```python
from build123d import *

# Parameters (mm, degrees)
F0_W        = 77.47
F0_H        = 19.05
F0_R        = 1.3890625
F0_W_2      = 52.07
F0_H_2      = 8.255
F0_W_3      = 7.62
F1_DEPTH    = 2.0574
F2_R        = 1.3890625
F2_W        = 46.99
F2_H        = 20.1539304107
F3_DEPTH    = 25.4
F4_T1_DEPTH = 2.0574


# Not quite as in the source:
# - a fillet or chamfer that OpenCascade refuses, or shapes differently, is made with other operations: its cross-section is extruded or revolved along the edge and cut away or added


with BuildPart() as f1:
    # F0 (on Top) → F1 (new body)
    with BuildSketch(Plane.XY):
        with Locations((29.845, 0)):
            Rectangle(F0_W, F0_H)
        with Locations((-4.2449974041, 0)):
            Circle(F0_R, mode=Mode.SUBTRACT)
        with Locations((-34.925, -13.6525)):
            Rectangle(F0_W_2, F0_H_2)
        with Locations((-34.925, 0)):
            Rectangle(F0_W_2, F0_H)
        with Locations((-64.77, 0)):
            Rectangle(F0_W_3, F0_H)
        with Locations((-64.6969974041, 0)):
            Circle(F0_R, mode=Mode.SUBTRACT)
        with Locations((-34.925, 13.6525)):
            Rectangle(F0_W_2, F0_H_2)
    extrude(amount=F1_DEPTH)

    # F2 (on face) → F3 (cut)
    with BuildSketch(Plane.XY.offset(2.0574)):
        Polygon((43.5640997417, 9.525), (68.58, 4.0749409236), (68.58, 9.525), align=None)
        Polygon((68.58, -9.525), (68.58, -4.0749409236), (43.5640997417, -9.525), align=None)
        with Locations((49.53, 0)):
            Circle(F2_R)
        with Locations((62.23, 0)):
            Circle(F2_R)
        with Locations((-35.5063436133, 0.5281241611)):
            Rectangle(F2_W, F2_H)
    extrude(amount=-F3_DEPTH, mode=Mode.SUBTRACT)

    # F4: fillet of radius 10.16 on 4 edges, made by hand

    # F4_s2 → F4_t1 (join)
    with BuildSketch(Plane.XY):
        with BuildLine():
            add(Edge.make_bspline(
                [(-22.1713436133, 10.6050893664), (-12.0113436133, 10.6050893664), (-12.0113436133, 0.4450893664)],
                knots=[0, 0, 0, 1, 1, 1], degree=2, weights=[1, 2.3333333333, 1]))
            Line((-12.0113436133, 0.4450893664), (-12.0113436133, 10.6050893664))
            Line((-12.0113436133, 10.6050893664), (-22.1713436133, 10.6050893664))
        make_face()
        with BuildLine():
            add(Edge.make_bspline(
                [(-48.8413436133, 10.6050893664), (-59.0013436133, 10.6050893664), (-59.0013436133, 0.4450893664)],
                knots=[0, 0, 0, 1, 1, 1], degree=2, weights=[1, 2.3333333333, 1]))
            Line((-59.0013436133, 0.4450893664), (-59.0013436133, 10.6050893664))
            Line((-59.0013436133, 10.6050893664), (-48.8413436133, 10.6050893664))
        make_face()
        with BuildLine():
            add(Edge.make_bspline(
                [(-59.0013436133, 0.6111589557), (-59.0013436133, -9.5488410443), (-48.8413436133, -9.5488410443)],
                knots=[0, 0, 0, 1, 1, 1], degree=2, weights=[1, 2.3333333333, 1]))
            Line((-48.8413436133, -9.5488410443), (-59.0013436133, -9.5488410443))
            Line((-59.0013436133, -9.5488410443), (-59.0013436133, 0.6111589557))
        make_face()
        with BuildLine():
            add(Edge.make_bspline(
                [(-22.1713436133, -9.5488410443), (-12.0113436133, -9.5488410443), (-12.0113436133, 0.6111589557)],
                knots=[0, 0, 0, 1, 1, 1], degree=2, weights=[1, 2.3333333333, 1]))
            Line((-12.0113436133, 0.6111589557), (-12.0113436133, -9.5488410443))
            Line((-12.0113436133, -9.5488410443), (-22.1713436133, -9.5488410443))
        make_face()
    extrude(amount=F4_T1_DEPTH)


solid = f1.part
```
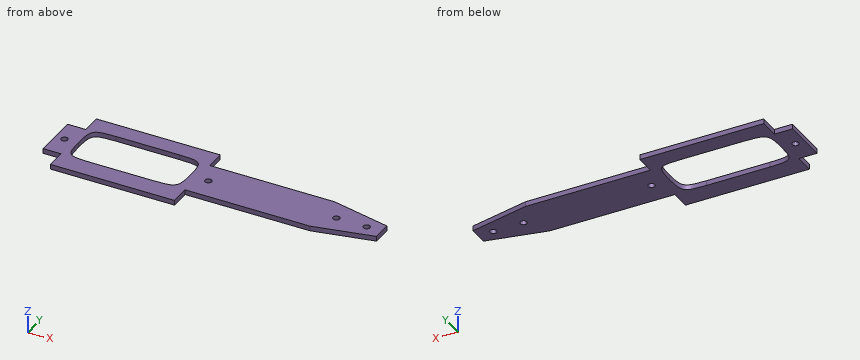
CAD build for the part. Positions are in the model's coordinates, mm. Round coordinates to 2 decimals unless told otherwise and drop trailing zeros. Write each loop counter-clockwise with the first axis right and the second up, starting at its lowest first coordinate (ties: lowest second). Pieces come first, ordered by that corner, then holes.
Item 1: Band-saw the part on A-A on x = -24. Write the cut outline in (y, z), then the cut area to 3 significant figures.
Filled in:
outline: (-17.78, 0) - (-9.55, 0) - (-9.55, 2.06) - (-17.78, 2.06) - close; (10.61, 0) - (17.78, 0) - (17.78, 2.06) - (10.61, 2.06) - close
area: 31.7 mm2
Item 2: Band-saw the part on B-B on z = 1.7. Give the number of separate pieces and of enclosed holes in the cut face, then the cut area to 3 significant figures.
Filled in:
separate pieces: 1
enclosed holes: 5
area: 2,400 mm2
Item 3: Band-saw the part on C-C on y = 14. Write the cut outline in (x, z).
Filled in:
outline: (-60.96, 0) - (-8.89, 0) - (-8.89, 2.06) - (-60.96, 2.06) - close
Item 4: Band-saw the part on D-D on x = -7. Write the cut outline in (y, z) (3 decimals).
Filled in:
outline: (-9.525, 0) - (9.525, 0) - (9.525, 2.057) - (-9.525, 2.057) - close
Item 5: Drop flat-ended pins along their axis: pin 1 Ø1 at (y, z) = (-11.5, 1) entering from +X; pin 2 Ø1.5 at (x, y) = (27.5, -10.5) entering from -Z; pin 3 Ø1 at (x, z) = (-64, 0.5) entering from +Y (3 decimals); pin 4 Ø0.6 at (x, z) = (16, 1.5) entering from -Y (3 decimals). Give the stop position or say it passes through.
Filled in:
pin 1: stops at x = -8.89
pin 2: passes through
pin 3: stops at y = 9.525
pin 4: stops at y = -9.525
Item 6: Drill centre lines: L1, parallel to Y at x = -28.5, z = 0.3; L2, parallel to Y at x = 40.5, z = 1.5 (3 decimals); L3, parallel to X at y = 12.5, z = 0.75. Where is each one in solid material? Low to high.
Filled in:
L1: y = -17.78 to -9.55, 10.61 to 17.78
L2: y = -9.525 to 9.525
L3: x = -60.96 to -8.89
